Part print with two shaded views. Sizes in mm from the minimum x, y, z corner. A direction names the side the tool comes from. Round coordinates to 2 decimals unless told otherwise and drop trailing zeros. Loops run counter-clockwise (first coordinate to the right, second up) from the corner with the lowest first, then second, coordinate; pieces in that order, holes last. Notation, with made-up numbers: (-24, 67) -> (10, 67) arc R16 ccw to (10, 89) -> close; hole circle Ø4 at (70, 81.25). An arc over 180 degrees is marked (long way). Use a Markdown table: item, result. Add a question column.
Item 1: Cut at C-C, the plane x = 25. List the corners of the cut face in (y, z).
Item 2: Which spindle directions (+Z, -Z, +X, -X, +Y, -Y) get a long thin tool onto all of the face, cutting with end or side? Do the marked faces 1 and 2. Say none if no direction does.
Item 3: Two-plate mould, pull along Y, no slides. Class the marked faces 3, 4, 5 and 6: pulls with the +Y half, pulls with the -Y half, needs draft (parallel to the pull), parting line crosses it, or undercut.
Item 4: Cut at B-B, the plane y = 50. List the corners of the cut face in (x, z).
Item 5: Cut at A-A, the plane z = 15. List the corners of the cut face in (x, y).
Item 6: Flat gauge pins, fed straight in: pin 1 (1.5 mm diameter, centred on x = 39, z = 28.5, fed in from -Y); pin 2 (1.5 mm diameter, centred on x = 30.5, z = 27, fed in from +Y); pin 3 (3 mm diameter, centred on x = 28.5, y = 17.5, fed in from +Z); pin 4 (12 mm diameter, centred on x = 28, y = 50.5, fed in from +Z). Where does each tip first touch, or does it go through?
Item 7: Cut at D-D, the plane y = 68.5. List the corners of the cut face in (x, z), plus the area to 3 significant figures.
Item 8: Probe line 1 (Y direction, x = 25, z = 23.75); line 2 (Y direction, x = 25, z = 19.5); line 3 (Y direction, x = 25, z = 21.75) (1 decimal). List the from-to ranges inside material, lowest first. Write a range as [from, to].
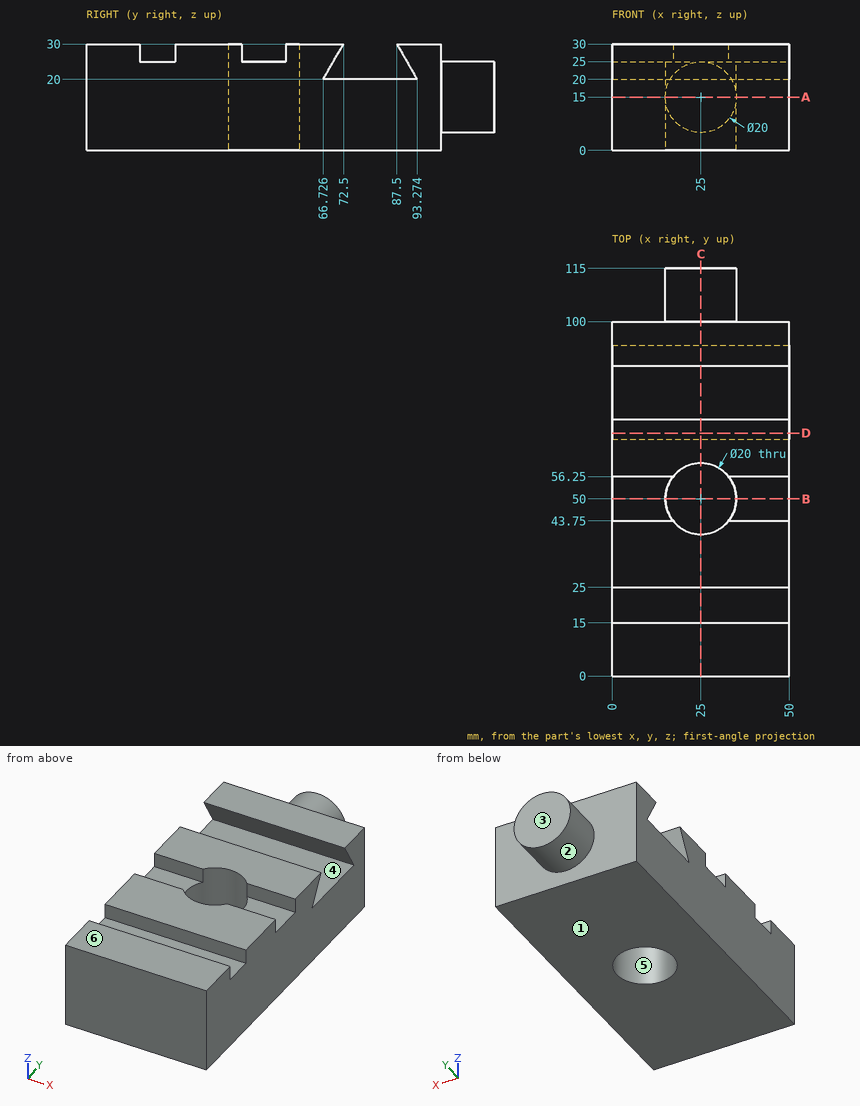
A:
| question | item | result |
|---|---|---|
| 1 | outline | (0, 0) -> (40, 0) -> (40, 30) -> (25, 30) -> (25, 25) -> (15, 25) -> (15, 30) -> (0, 30) -> close; (60, 0) -> (100, 0) -> (100, 5) -> (115, 5) -> (115, 25) -> (100, 25) -> (100, 30) -> (87.5, 30) -> (93.27, 20) -> (66.73, 20) -> (72.5, 30) -> (60, 30) -> close |
| 2 | face 1 | -Z, +X, -X, +Y, -Y |
| 2 | face 2 | +Y |
| 3 | face 3 | pulls with the +Y half |
| 3 | face 4 | undercut |
| 3 | face 5 | undercut |
| 3 | face 6 | needs draft |
| 4 | outline | (0, 0) -> (15, 0) -> (15, 25) -> (0, 25) -> close; (35, 0) -> (50, 0) -> (50, 25) -> (35, 25) -> close |
| 5 | outline | (0, 0) -> (50, 0) -> (50, 100) -> (35, 100) -> (35, 115) -> (15, 115) -> (15, 100) -> (0, 100) -> close; hole circle Ø20 at (25, 50) |
| 6 | pin 1 | stops at y = 0 |
| 6 | pin 2 | stops at y = 100 |
| 6 | pin 3 | stops at z = 25 |
| 6 | pin 4 | passes through |
| 7 | outline | (0, 0) -> (50, 0) -> (50, 20) -> (0, 20) -> close; (0, 23.07) -> (50, 23.07) -> (50, 30) -> (0, 30) -> close |
| 7 | area | 1,350 mm^2 |
| 8 | line 1 | y = [0, 40], [60, 68.89], [91.11, 115] |
| 8 | line 2 | y = [0, 40], [60, 115] |
| 8 | line 3 | y = [0, 40], [60, 67.7], [92.3, 115] |
